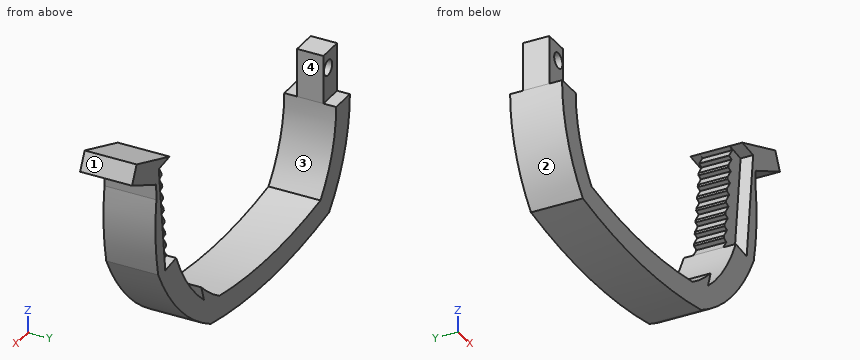
```python
from build123d import *

# Parameters (mm, degrees)
F1_DEPTH = 10.15
F2_W     = 1.8519068835
F2_H     = 21.5889067106
F2_W_2   = 2.4580931165
F3_DEPTH = 4
F5_DEPTH = 7.6929068835
F6_W     = 5
F6_H     = 5.15
F7_DEPTH = 9.5
F8_R     = 1.5
F9_DEPTH = 7.651


with BuildPart() as f1:
    # F0 (on Front) → F1 (new body)
    with BuildSketch(Plane.XZ):
        with BuildLine():
            ThreePointArc((-18.5, -15.6787953926), (-22.7673477806, -8.35), (-24.2502499979, 0))
            Line((-24.2502499979, 0), (-29.2502499979, 0))
            ThreePointArc((-29.2502499979, 0), (-27.2813970489, -10.55), (-21.6398876928, -19.6797455671))
            ThreePointArc((-21.6398876928, -19.6797455671), (0, -21.8765954826), (21.6398876928, -19.6797455671))
            ThreePointArc((21.6398876928, -19.6797455671), (32.7568623734, -11.3164689916), (40.8481571207, 0))
            ThreePointArc((40.8481571207, 0), (41.8214250715, 7.632604285), (41.4990372956, 15.3202544329))
            Line((41.4990372956, 15.3202544329), (41.5767828027, 18.3806335645))
            Line((41.5767828027, 18.3806335645), (50.389803946, 22.7065682411))
            Line((50.389803946, 22.7065682411), (48.7227849662, 26.10270679))
            Line((48.7227849662, 26.10270679), (36.6513244808, 21.4579887688))
            Line((36.6513244808, 21.4579887688), (34.277380304, 0))
            ThreePointArc((34.277380304, 0), (29.9691571864, -7.3960863272), (24.0930236738, -13.6197455671))
            Line((24.0930236738, -13.6197455671), (25.0645451381, -10.5997455671))
            ThreePointArc((25.0645451381, -10.5997455671), (21.92981042, -13.3299594699), (18.5, -15.6787953926))
            ThreePointArc((18.5, -15.6787953926), (0, -17.3512801115), (-18.5, -15.6787953926))
        make_face()
    extrude(amount=F1_DEPTH)

    # F2 (on face) → F3 (cut)
    with BuildSketch(Plane(origin=(33.8629158132, 0, -3.7463283568), x_dir=(0, -1, 0), z_dir=(-0.9939358698, 0, 0.1099612967))):
        with Locations((0.9259534418, 14.5636385419)):
            Rectangle(F2_W, F2_H)
        with Locations((8.9209534418, 14.5636385419)):
            Rectangle(F2_W_2, F2_H)
    extrude(amount=-F3_DEPTH, mode=Mode.SUBTRACT)

    # F4 (on face) → F5 (cut, through all)
    with BuildSketch(Plane.XZ.offset(7.6919068835)):
        Polygon((34.4986446734, 2), (34.277380304, 0), (35.4295624031, 1.6347710575), align=None)
        Polygon((36.2071527972, 17.4431382552), (36.4265479737, 19.4262426935), (36.379591068, 19.4431382552), align=None)
        Polygon((35.9315717956, 14.9521723361), (36.1512704613, 16.9380200021), (36.1125353235, 16.9521723361), align=None)
        Polygon((35.6560050027, 12.4613348501), (35.8756791772, 14.4469611397), (35.8362903057, 14.4613348501), align=None)
        Polygon((35.3804528293, 9.9706295076), (35.6001020466, 11.9560302114), (35.5600452879, 11.9706295076), align=None)
        Polygon((35.2964822054, 9.4777310046), (35.1046580216, 7.4777310046), (35.324757133, 9.4671982825), align=None)
        Polygon((35.0074181049, 6.9872777462), (34.8291337367, 4.9872777462), (35.0487360064, 6.9722540912), align=None)
        Polygon((34.7311730871, 4.4969679349), (34.5536253217, 2.4969679349), (34.7732012529, 4.4817062071), align=None)
        Polygon((37.0518071993, 16.6089984104), (36.1512704613, 16.9380200021), (35.9315717956, 14.9521723361), align=None)
        Polygon((36.7756964321, 14.1185285934), (35.8756791772, 14.4469611397), (35.6560050027, 12.4613348501), align=None)
        Polygon((36.4995883451, 11.628198721), (35.6001020466, 11.9560302114), (35.3804528293, 9.9706295076), align=None)
        Polygon((35.324757133, 9.4671982825), (35.1046580216, 7.4777310046), (36.2335759695, 9.128653252), align=None)
        Polygon((35.0487360064, 6.9722540912), (34.8291337367, 4.9872777462), (35.9472190993, 6.645555504), align=None)
        Polygon((34.7732012529, 4.4817062071), (34.5536253217, 2.4969679349), (35.6711189912, 4.1556444852), align=None)
        Polygon((37.5822422105, 21.0927598263), (36.6513244808, 21.4579887688), (36.4300601114, 19.4579887688), align=None)
        Polygon((37.320535459, 19.104577104), (36.4265479737, 19.4262426935), (36.2071527972, 17.4431382552), align=None)
    extrude(amount=-F5_DEPTH, mode=Mode.SUBTRACT)

    # F6 (on face) → F7 (join)
    with BuildSketch(Plane.XY):
        with Locations((-26.7502499979, -5.075)):
            Rectangle(F6_W, F6_H)
    extrude(amount=F7_DEPTH)

    # F8 (on face) → F9 (cut, through all)
    with BuildSketch(Plane(origin=(0, -2.5, 0), x_dir=(-1, 0, 0), z_dir=(0, 1, 0))):
        with Locations((25.9502499979, 6.3)):
            Circle(F8_R)
    extrude(amount=-F9_DEPTH, mode=Mode.SUBTRACT)


solid = f1.part
```
Build history of the part. All positions in model axes, mm. Face numbers are marked on the shaded views. Coordinates: 2 decimals unless noted, no trailing zeros. Order: outer loops, then holes, each group sorted by start corner. A loop starts at its lowest first (then second) coordinate and runs counter-clockwise, first axis right, second up.
Item 1: Saw through at B-B on x = 31.5. List the corners of the cut face in (y, z), then the cut area to 3 significant figures.
Filled in:
outline: (-10.15, -12.56) - (0, -12.56) - (0, -5.19) - (-10.15, -5.19) - close
area: 74.8 mm2
Item 2: Drop flat-ended pins along their axis: pin 1 Ø2.5 at (x, y) = (-26.5, -5) entering from +Z; pin 2 Ø2.5 at (x, z) = (-27.5, 6.5) entering from +Y; pin 3 Ø1.5 at (y, z) = (-6, -4) entering from +X; pin 4 Ø6 at (x, z) = (-19.5, 10) entering from +Y. Give the stop position or say it passes through.
Filled in:
pin 1: stops at z = 9.5
pin 2: stops at y = -2.5
pin 3: stops at x = 39.04
pin 4: passes through
Item 3: Mould opens along X. For the marked faces 1, 2, 3 and 4 say: released by +X, released by -X, zero draft, split by the parting line, or undercut.
Filled in:
face 1: released by +X
face 2: released by -X
face 3: undercut
face 4: undercut
Item 4: Saw through at A-A on z = -8. List the corners of the cut face in (x, y), then the cut area to 3 significant figures.
Filled in:
outline: (-28.13, -10.15) - (-22.89, -10.15) - (-22.89, 0) - (-28.13, 0) - close; (29.51, -10.15) - (35.69, -10.15) - (35.69, 0) - (29.51, 0) - close
area: 116 mm2
Item 5: Saw through at C-C on x = -11. List the corners of the cut face in (y, z).
Filled in:
outline: (-10.15, -21.31) - (0, -21.31) - (0, -16.76) - (-10.15, -16.76) - close
Item 6: Drill centre lines: L1, parallel to Z at x = 35.5, y = -6.25; L2, parallel to X at y = -4.25, z = -4.5; L3, parallel to X at y = -1, z = -9.5. Where is each one in solid material? Low to high.
Filled in:
L1: z = -8.24 to 3.9, 4.22 to 5.98, 6.81 to 8.06, 9.4 to 10.15
L2: x = -28.9 to -23.83, 31.93 to 38.24
L3: x = -27.66 to -22.31, 28.27 to 34.44
